The model under review builds one solid part; all positions refer to its coordinate system, in mm. Coordinates: 2 decimals unless noted, no trailing zeros. Order: outer loops, then holes, each group sorted by start corner. A loop starts at its lowest first (then second) coordinate and runs counter-clockwise, first axis right, second up. Notation, with made-up numbers: (-7.75, 51.5) - (42.25, 51.5) arc R28 cw to (42.25, 81.5) - close; hole circle Ø9 at (76.5, 49). An arc over 180 degrees is marked (long way). Answer in a Markdown table with one row per item.
```python
from build123d import *

# Parameters (mm, degrees)
SKETCH1_W           = 82
SKETCH1_H           = 70
SKETCH1_R           = 14.295
SKETCH1_R_2         = 2.6
BOSS_EXTRUDE1_DEPTH = 6.35
CHAMFER1_SIZE       = 15


with BuildPart() as part:
    # Sketch1 → Boss-Extrude1 (new body)
    with BuildSketch(Plane(origin=(0, 0, 0), x_dir=(0, 0, -1), z_dir=(1, 0, 0))):
        Rectangle(SKETCH1_W, SKETCH1_H)
        Circle(SKETCH1_R, mode=Mode.SUBTRACT)
        with Locations((-31, 0)):
            Circle(SKETCH1_R_2, mode=Mode.SUBTRACT)
        with Locations((31, 0)):
            Circle(SKETCH1_R_2, mode=Mode.SUBTRACT)
    extrude(amount=BOSS_EXTRUDE1_DEPTH)

    # Chamfer1
    chamfer1_edges = [part.edges().sort_by_distance(p)[0] for p in [
        (3.175, 35, 41),
        (3.175, 35, -41),
        (3.175, -35, -41),
        (3.175, -35, 41),
    ]]
    chamfer(chamfer1_edges, length=CHAMFER1_SIZE)


solid = part.part
```
Item 1: To check wall thickness, follow line 1 (Y direction, x = 4.25, z = 0) (3 decimals); line 2 (Z direction, x = 3.5, y = 5); line 3 (Y direction, x = 1.5, z = 31). State the ranges of each line that lie inside material, in increasing order. Write a range as from..to.
Check values:
| item | result |
|---|---|
| line 1 | -35..-14.295, 14.295..35 |
| line 2 | -41..-13.39, 13.39..41 |
| line 3 | -30..-2.6, 2.6..30 |
Item 2: We need section C-C, the plane y = 0. Write out the cut boundary in (x, z) (3 decimals).
Check values:
| item | result |
|---|---|
| outline | (0, -41) - (6.35, -41) - (6.35, -33.6) - (0, -33.6) - close; (0, -28.4) - (6.35, -28.4) - (6.35, -14.295) - (0, -14.295) - close; (0, 14.295) - (6.35, 14.295) - (6.35, 28.4) - (0, 28.4) - close; (0, 33.6) - (6.35, 33.6) - (6.35, 41) - (0, 41) - close |
Item 3: We need section B-B, the plane x = 5. Write out the cut boundary in (y, z) (3 decimals), then the cut area to 3 significant figures.
Check values:
| item | result |
|---|---|
| outline | (-35, -26) - (-20, -41) - (20, -41) - (35, -26) - (35, 26) - (20, 41) - (-20, 41) - (-35, 26) - close; hole circle Ø28.59 at (0, 0); hole circle Ø5.2 at (0, -31); hole circle Ø5.2 at (0, 31) |
| area | 4,610 mm^2 |
Item 4: Mouldability with a two-part tool opening along Z and no side actions: class faces 1 (the face through (3.1, 0.1, 33.6)), 2 (the face through (3.1, 0.1, -28.4)), 3 (the face through (3, 35, 0)), 4 (the face through (3, -28, 33)) as +Z half, -Z half, draft (parallel to the pull), parting line (faces both ways), or undercut.
Check values:
| item | result |
|---|---|
| face 1 | undercut |
| face 2 | undercut |
| face 3 | draft |
| face 4 | +Z half |
Item 5: We need section A-A, the plane z = 0. Write out the cut boundary in (x, y) (3 decimals), then the cut area to 3 significant figures.
Check values:
| item | result |
|---|---|
| outline | (0, -35) - (6.35, -35) - (6.35, -14.295) - (0, -14.295) - close; (0, 14.295) - (6.35, 14.295) - (6.35, 35) - (0, 35) - close |
| area | 263 mm^2 |
Item 6: We need section D-D, the plane y = -12. Write out the cut boundary in (x, z), then the cut area to 3 significant figures.
Check values:
| item | result |
|---|---|
| outline | (0, -41) - (6.35, -41) - (6.35, -7.77) - (0, -7.77) - close; (0, 7.77) - (6.35, 7.77) - (6.35, 41) - (0, 41) - close |
| area | 422 mm^2 |
